For this review, take the finished solid that the model builds, in its own axes (mm). Coordinates: 2 decimals unless noted, no trailing zeros. Write each loop counter-clockwise with the first axis right and the second up, starting at its lowest first coordinate (ties: lowest second). Pieces come first, ordered by that corner, then holes.
```python
from build123d import *

# Parameters (mm, degrees)
BOSS_EXTRUDE2_DEPTH      = 514
BOSS_EXTRUDE2_DEPTH_BACK = 40
CUT_EXTRUDE1_DEPTH       = 3636.875029428
CUT_EXTRUDE1_DEPTH_BACK  = 3636.875029428


with BuildPart() as part:
    # Sketch1 → Boss-Extrude2 (new, two sides: drawn at the far end of the back side and taken through both)
    with BuildSketch(Plane.XY.offset(-BOSS_EXTRUDE2_DEPTH_BACK)):
        with BuildLine():
            Line((14.404810003, 5.178419046), (14.404810003, 14.708419046))
            Line((14.404810003, 14.708419046), (24.404810003, 14.708419046))
            Line((24.404810003, 14.708419046), (24.404810003, 19.708419046))
            Line((24.404810003, 19.708419046), (-17.916389143, 19.708419046))
            Line((-17.916389143, 19.708419046), (-21.938692577, -22.421202033))
            Line((-21.938692577, -22.421202033), (-16.961326395, -22.896413454))
            Line((-16.961326395, -22.896413454), (-16.010903554, -12.941681091))
            Line((-16.010903554, -12.941681091), (-6.524043612, -13.847434058))
            ThreePointArc((-6.524043612, -13.847434058), (0, 0), (14.404810003, 5.178419046))
        make_face()
    extrude(amount=BOSS_EXTRUDE2_DEPTH + BOSS_EXTRUDE2_DEPTH_BACK)

    # Sketch2 → Cut-Extrude1 (cut, two sides: drawn at the far end of the back side and taken through both)
    with BuildSketch(Plane(origin=(-738.20187256, 812.038169561, 3415.561100518), x_dir=(-0.955618514406147, 0, -0.2946069498911878), z_dir=(0.0908241663548398, 0.9512926552232807, -0.29460694989118763)).offset(-CUT_EXTRUDE1_DEPTH_BACK)):
        Polygon((69.88483537, -3135.609871351), (246.824126872, -3135.609871351), (167.605357186, -3034.434147623), align=None)
        Polygon((236.262195777, -3561.307235785), (313.780261045, -3654.403893751), (393.908665817, -3561.307235785), align=None)
    extrude(amount=CUT_EXTRUDE1_DEPTH + CUT_EXTRUDE1_DEPTH_BACK, mode=Mode.SUBTRACT)


solid = part.part
```
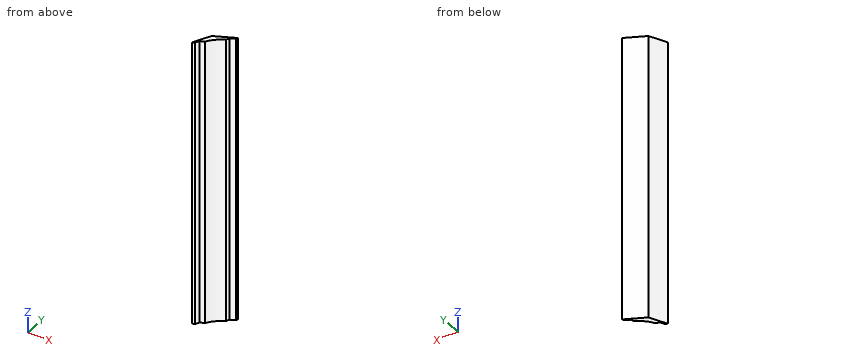
Q1. Add section A-A (z = 135). State the section outline as (x, y) points.
Ans:
outline: (-21.94, -22.42) - (-16.96, -22.9) - (-16.01, -12.94) - (-6.52, -13.85) arc R20 cw to (14.4, 5.18) - (14.4, 14.71) - (24.4, 14.71) - (24.4, 19.71) - (-17.92, 19.71) - close
Q2. Add section C-C (y = -8.5). State the section outline as (x, z) points, then the cut area to 3 significant figures.
Ans:
outline: (-20.61, -2.46) - (-5.53, 2.19) - (-5.53, 470.46) - (-20.61, 465.81) - close
area: 7,060 mm2
Q3. Clearance check with flat-ended pins moving along their axes: pin 1 Ø5 at (x, y) = (-11.5, -7.5) entering from +Z; pin 2 Ø3 at (y, z) = (12, 130.5) entering from +X; pin 3 Ø3 at (y, z) = (-9.5, 370) entering from +X. State where each tip first meets the part, or that it passes through.
Ans:
pin 1: stops at z = 469.43
pin 2: stops at x = 14.4
pin 3: stops at x = -5.36
Q4. Add section B-B (x = -12). State the section outline as (y, z) points.
Ans:
outline: (-13.32, 1.83) - (19.71, -9.38) - (19.71, 458.9) - (-13.32, 470.1) - close
Q5. For probe 1 along Y at (x, z) = (20, 72.5); probe 2 along X at (y, z) = (-3, 141); probe 3 along X at (y, z) = (-9.5, 157.5), list the stretches that pass through material, from the lowest coordinate up.
Ans:
probe 1: y = 14.71 to 19.71
probe 2: x = -20.08 to -2.7
probe 3: x = -20.71 to -5.83
